Could you check a few things on this model? Use its own coordinates, in mm. Face numbers are marked on the shaded views. A direction names the side the tool comes from. Give positions to 0.01 mm unless a question says otherwise; leave off trailing zeros. Write each loop counter-clockwise with the first axis right and the second up, starting at its lowest first coordinate (ties: lowest second). Pieces come first, ordered by that corner, then holes. Notation, with made-up numbers: (-37, 35.25) - (-16, 35.25) arc R32 cw to (-16, 72.25) - close; hole circle Ø7 at (14.25, 50). An arc over 180 degrees is marked (long way). Answer in a Markdown table with one row per item.
from build123d import *

# Parameters (mm, degrees)
F0_R     = 10
F1_DEPTH = 6
F5_R     = 0.5
F6_DEPTH = 12.001


with BuildPart() as f1:
    # F0 (on Front) → F1 (new body, symmetric)
    with BuildSketch(Plane.XZ):
        Circle(F0_R)
    extrude(amount=F1_DEPTH, both=True)

    # F3 (on Right) → F4 (revolve, cut)
    with BuildSketch(Plane.YZ):
        with BuildLine():
            Line((3.75, 10), (-3.75, 10))
            Line((-3.75, 10), (-3.75, 7.5))
            ThreePointArc((-3.75, 7.5), (-2.724874, 5.025126), (-0.25, 4))
            Line((-0.25, 4), (0.25, 4))
            ThreePointArc((0.25, 4), (2.724874, 5.025126), (3.75, 7.5))
            Line((3.75, 7.5), (3.75, 10))
        make_face()
    revolve(axis=Axis((0, -0.154715, 0), (0, -1, 0)), mode=Mode.SUBTRACT)

    # F5 (on face) → F6 (cut, through all)
    with BuildSketch(Plane(origin=(0, 6, 0), x_dir=(-1, 0, 0), z_dir=(0, 1, 0))):
        Circle(F5_R)
    extrude(amount=-F6_DEPTH, mode=Mode.SUBTRACT)


solid = f1.part
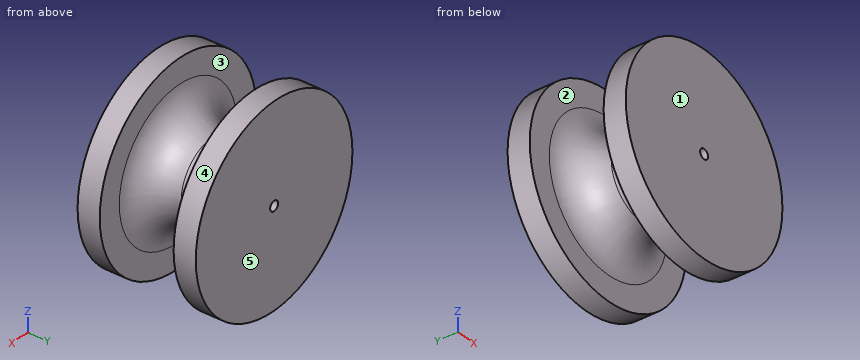
1) Imagine slicing it at D-D (x = -8.25). List the corners of the cut face in (y, z) for me.
Check values:
| item | result |
|---|---|
| outline | (-6, -5.65) - (-3.75, -5.65) - (-3.75, 5.65) - (-6, 5.65) - close; (3.75, -5.65) - (6, -5.65) - (6, 5.65) - (3.75, 5.65) - close |
2) If I drill on line 1 (Y direction, x = 7.25, z = -5); line 2 (Z direction, x = 0, y = -2.5), over which ranges is the centre line in solid material (lowest first)?
Check values:
| item | result |
|---|---|
| line 1 | y = -6 to -3.75, 3.75 to 6 |
| line 2 | z = -4.82 to -0.5, 0.5 to 4.82 |
3) We'd pull the mould along Y, two halves only. Please class the marked faces 3, 4 and 5: +Y half, -Y half, draft (parallel to the pull), parting line (faces both ways), or undercut.
Check values:
| item | result |
|---|---|
| face 3 | undercut |
| face 4 | draft |
| face 5 | +Y half |
4) Imagine slicing it at A-A (x = 0). List the corners of the cut face in (y, z) for me.
Check values:
| item | result |
|---|---|
| outline | (-6, -10) - (-3.75, -10) - (-3.75, -7.5) arc R3.5 cw to (-0.25, -4) - (0.25, -4) arc R3.5 cw to (3.75, -7.5) - (3.75, -10) - (6, -10) - (6, -0.5) - (-6, -0.5) - close; (-6, 0.5) - (6, 0.5) - (6, 10) - (3.75, 10) - (3.75, 7.5) arc R3.5 cw to (0.25, 4) - (-0.25, 4) arc R3.5 cw to (-3.75, 7.5) - (-3.75, 10) - (-6, 10) - close |
5) Imagine slicing it at B-B (z = 0). List the corners of the cut face in (x, y) for me, then the cut area to 3 significant figures.
Check values:
| item | result |
|---|---|
| outline | (-10, -6) - (-0.5, -6) - (-0.5, 6) - (-10, 6) - (-10, 3.75) - (-7.5, 3.75) arc R3.5 cw to (-4, 0.25) - (-4, -0.25) arc R3.5 cw to (-7.5, -3.75) - (-10, -3.75) - close; (0.5, -6) - (10, -6) - (10, -3.75) - (7.5, -3.75) arc R3.5 cw to (4, -0.25) - (4, 0.25) arc R3.5 cw to (7.5, 3.75) - (10, 3.75) - (10, 6) - (0.5, 6) - close |
| area | 149 mm2 |
6) Imagine slicing it at C-C (y = -4). List the corners of the cut face in (x, z) for me.
Check values:
| item | result |
|---|---|
| outline | circle Ø20 at (0, 0); hole circle Ø1 at (0, 0) |
7) Will these pins go through, and if not, where does the flat tip stop? P1, Ø2, axis at x = 1.5, y = 0.5, coming from the +Z side; P2, Ø4, axis at x = -3, y = 1, coming from the +Z side; P3, Ø1, axis at y = -2, z = 4.5, coming from the -X side.
Check values:
| item | result |
|---|---|
| P1 | stops at z = 4.06 |
| P2 | stops at z = 4.65 |
| P3 | stops at x = -2.22 |
8) On a 3-axis mill with a long thin cutter (end or side, diameter ignored), from which of +Z, -Z, +X, -X, +Y, -Y can I reach the whole of each face in a straight line? I mean the marked faces 1 and 2. Say none if no direction works.
Check values:
| item | result |
|---|---|
| face 1 | +Z, -Z, +X, -X, -Y |
| face 2 | none |
